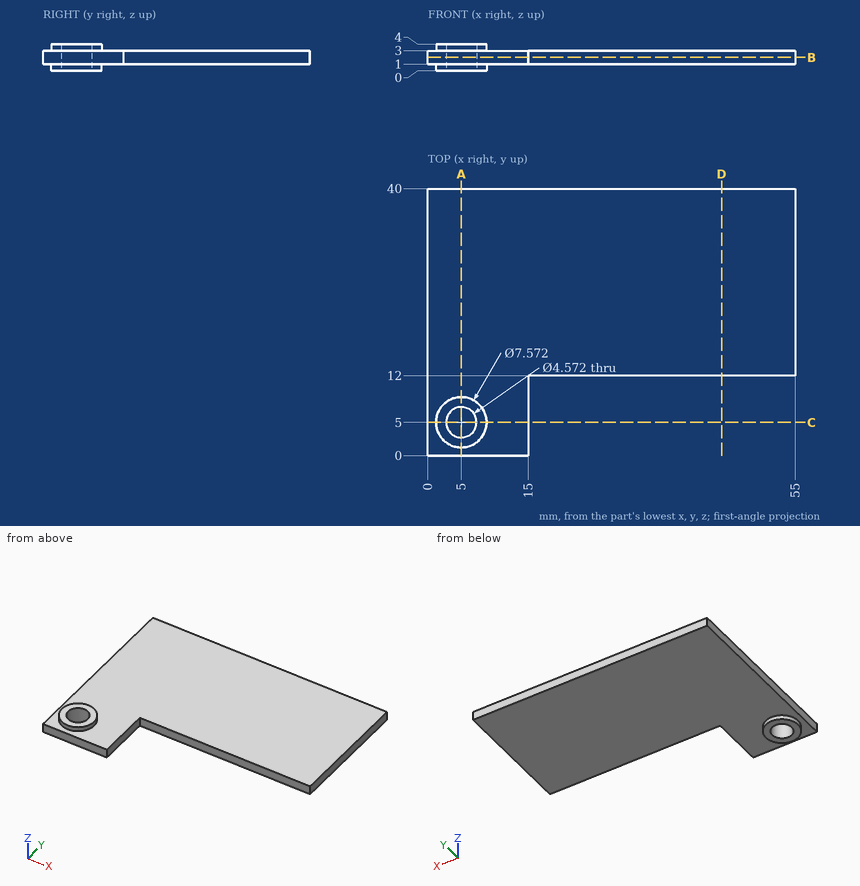
Could you check a few things on this drawing? It's one solid part, dimensions in mm from its lowest x, y, z. Round coordinates to 2 decimals unless told otherwise and drop trailing zeros. Order: outer loops, then holes, each group sorted by start corner. A loop starts at its lowest first (then second) coordinate and runs counter-clockwise, first axis right, second up.
(1) I'm going to push flat-ended pins straight in: pin 1 (12 mm diameter, centred on x = 22.5, y = 20.5, fed in from -Z); pin 2 (0.6 mm diameter, centred on x = 34.5, z = 2, fed in from -Y); pin 3 (8 mm diameter, centred on x = 46.5, y = 35, fed in from +Z). Where does each tip first touch, or does it pass through?
Response values:
pin 1: stops at z = 1
pin 2: stops at y = 12
pin 3: stops at z = 3
(2) Imagine slicing it at D-D (x = 44). Write out the boundary of the cut face in (y, z), plus the area to 3 significant figures.
Response values:
outline: (12, 1) - (40, 1) - (40, 3) - (12, 3) - close
area: 56.0 mm2
(3) Imagine slicing it at A-A (x = 5). Write out the boundary of the cut face in (y, z).
Response values:
outline: (0, 1) - (1.21, 1) - (1.21, 0) - (2.71, 0) - (2.71, 4) - (1.21, 4) - (1.21, 3) - (0, 3) - close; (7.29, 0) - (8.79, 0) - (8.79, 1) - (40, 1) - (40, 3) - (8.79, 3) - (8.79, 4) - (7.29, 4) - close
(4) Imagine slicing it at C-C (y = 5). Write out the boundary of the cut face in (x, z).
Response values:
outline: (0, 1) - (1.21, 1) - (1.21, 0) - (2.71, 0) - (2.71, 4) - (1.21, 4) - (1.21, 3) - (0, 3) - close; (7.29, 0) - (8.79, 0) - (8.79, 1) - (15, 1) - (15, 3) - (8.79, 3) - (8.79, 4) - (7.29, 4) - close
(5) Imagine slicing it at B-B (z = 2). Write out the boundary of the cut face in (x, y), plus the area to 3 significant figures.
Response values:
outline: (0, 0) - (15, 0) - (15, 12) - (55, 12) - (55, 40) - (0, 40) - close; hole circle Ø4.57 at (5, 5)
area: 1,700 mm2
(6) Please list where these lines run through material, in increasing order: line 1 along Y through (x, z) = (5, 2.55); line 2 along X through (y, z) = (2.5, 2.7); line 3 along Z through (x, y) = (37.5, 34.5).
Response values:
line 1: y = 0 to 2.71, 7.29 to 40
line 2: x = 0 to 15
line 3: z = 1 to 3
